from build123d import *

# Parameters (mm, degrees)
SKETCH_1_R           = 3
SKETCH_1_R_2         = 1.2
EXTRUDE_1_DEPTH      = 4.5
EXTRUDE_2_DEPTH      = 4.5
EXTRUDE_2_DEPTH_BACK = 2.5
SKETCH_2_R           = 1.2
FILLET_1_R           = 8
CUT_EXTRUDE_1_REACH  = 62.544
SKETCH_3_R           = 3.421397557
FILLET_2_R           = 3
CUT_EXTRUDE_2_DEPTH  = 1.7
FILLET_START         = 2
FILLET_3_DEPTH       = 2.5


with BuildPart() as part:
    # 草图1 → 凸台-拉伸1 (new body)
    with BuildSketch(Plane.XY):
        Polygon((-12.5, 0), (-18.5, 0), (-18.5, 42.034916596), (0, 60.534916596), (18.5, 42.034916596), (18.5, 0), (12.5, 0), (12.5, 35), (-12.5, 35), align=None)
        with Locations((0, 50.421397557)):
            Circle(SKETCH_1_R, mode=Mode.SUBTRACT)
        with Locations((-15.5, 5)):
            Circle(SKETCH_1_R_2, mode=Mode.SUBTRACT)
        with Locations((-15.5, 26)):
            Circle(SKETCH_1_R_2, mode=Mode.SUBTRACT)
        with Locations(Location((15.5, 5, 0), (0, 0, 180))):
            Circle(SKETCH_1_R_2, mode=Mode.SUBTRACT)
        with Locations(Location((15.5, 26, 0), (0, 0, 180))):
            Circle(SKETCH_1_R_2, mode=Mode.SUBTRACT)
    extrude(amount=EXTRUDE_1_DEPTH)

    # 草图2 → 凸台-拉伸2 (add, two sides: drawn at the far end of the back side and taken through both)
    # profile 1 of 2: a face of its own
    with BuildSketch(Plane.XY.offset(4.5).offset(-EXTRUDE_2_DEPTH_BACK)):
        with BuildLine():
            Line((17.5, 47), (3.906515802, 47))
            ThreePointArc((3.906515802, 47), (5.192959363, 50.421397557), (3.906515802, 53.842795113))
            Line((3.906515802, 53.842795113), (17.5, 53.842795113))
            Line((17.5, 53.842795113), (17.5, 47))
        make_face()
        with Locations(Location((12.5, 50.421397557, 0), (0, 0, 180))):
            Circle(SKETCH_2_R, mode=Mode.SUBTRACT)
    # profile 2 of 2: a face of its own
    with BuildSketch(Plane.XY.offset(4.5).offset(-EXTRUDE_2_DEPTH_BACK)):
        with BuildLine():
            Line((-17.5, 47), (-17.5, 53.842795113))
            Line((-17.5, 53.842795113), (-3.906515802, 53.842795113))
            ThreePointArc((-3.906515802, 53.842795113), (-5.192959363, 50.421397557), (-3.906515802, 47))
            Line((-3.906515802, 47), (-17.5, 47))
        make_face()
        with Locations((-12.5, 50.421397557)):
            Circle(SKETCH_2_R, mode=Mode.SUBTRACT)
    extrude(amount=EXTRUDE_2_DEPTH + EXTRUDE_2_DEPTH_BACK)

    # 圆角1
    fillet_1_edges = [part.edges().sort_by_distance(p)[0] for p in [
        (-18.5, 42.034916596, 2.25),
        (0, 60.534916596, 2.25),
        (18.5, 42.034916596, 2.25),
    ]]
    fillet(fillet_1_edges, radius=FILLET_1_R)

    # 草图3 → 切除-拉伸1 (cut, up to next)
    with BuildSketch(Plane(origin=(0, 0, 2), x_dir=(-1, 0, 0), z_dir=(0, 0, -1)), mode=Mode.PRIVATE) as cut_extrude_1_sk1:
        with Locations((-12.5, 50.421397557)):
            Circle(SKETCH_3_R)
    cut_extrude_1_tool1 = extrude(cut_extrude_1_sk1.sketch, amount=CUT_EXTRUDE_1_REACH, mode=Mode.PRIVATE) & part.part
    # 草图3 → 切除-拉伸1 (cut, up to next)
    with BuildSketch(Plane(origin=(0, 0, 2), x_dir=(-1, 0, 0), z_dir=(0, 0, -1)), mode=Mode.PRIVATE) as cut_extrude_1_sk2:
        with Locations((12.5, 50.421397557)):
            Circle(SKETCH_3_R)
    cut_extrude_1_tool2 = extrude(cut_extrude_1_sk2.sketch, amount=CUT_EXTRUDE_1_REACH, mode=Mode.PRIVATE) & part.part
    add(cut_extrude_1_tool1.solids().sort_by_distance((12.5, 50.421398, 2))[0], mode=Mode.SUBTRACT)
    add(cut_extrude_1_tool2.solids().sort_by_distance((-12.5, 50.421398, 2))[0], mode=Mode.SUBTRACT)

    # 圆角2
    fillet_2_edges = [part.edges().sort_by_distance(p)[0] for p in [
        (9.202203088, 51.332713509, 1),
        (-9.202203088, 51.332713509, 1),
        (-6.692121483, 53.842795113, 3.25),
        (-17.5, 47, 5.5),
        (-5.192959363, 50.421397557, 9),
        (-17.5, 53.842795113, 5.5),
        (6.692121483, 53.842795113, 3.25),
        (17.5, 53.842795113, 5.5),
        (5.192959363, 50.421397557, 9),
        (17.5, 47, 5.5),
    ]]
    fillet(fillet_2_edges, radius=FILLET_2_R)

    # 草图4 → 切除-拉伸2 (cut)
    with BuildSketch(Plane.XY.offset(9)):
        Polygon((0, 46.899022366), (43.079074711, 50.891584803), (0, 53.943772747), (-43.079074711, 50.891584803), align=None)
    extrude(amount=-CUT_EXTRUDE_2_DEPTH, mode=Mode.SUBTRACT)

    # 圆角3: read off the stored shape, not the designer's step
    # 圆角3 outline → 圆角3 (add)
    with BuildSketch(Plane.XY.offset(FILLET_START)):
        with BuildLine():
            ThreePointArc((17.623806552, 42.361452624), (16.757691875, 45.600251323), (17.294803574, 48.909553768))
            ThreePointArc((17.294803574, 48.909553768), (16.192433353, 47.52297167), (14.5, 47))
            Line((14.5, 47), (13.534916596, 47))
            Line((13.534916596, 47), (16.156854249, 44.378062347))
            ThreePointArc((16.156854249, 44.378062347), (16.969389563, 43.42726788), (17.623806552, 42.361452624))
        make_face()
        with BuildLine():
            ThreePointArc((-14.5, 47), (-16.192433353, 47.52297167), (-17.294803574, 48.909553768))
            ThreePointArc((-17.294803574, 48.909553768), (-16.757691875, 45.600251323), (-17.623806552, 42.361452624))
            ThreePointArc((-17.623806552, 42.361452624), (-16.969389563, 43.42726788), (-16.156854249, 44.378062347))
            Line((-16.156854249, 44.378062347), (-13.534916596, 47))
            Line((-13.534916596, 47), (-14.5, 47))
        make_face()
    extrude(amount=FILLET_3_DEPTH)


solid = part.part
CAD build for the part. Positions are in the model's coordinates, mm. A direction names the side the tool comes from. Round coordinates to 2 decimals unless told otherwise and drop trailing zeros. Loops run counter-clockwise (first coordinate to the right, second up) from the corner with the lowest first, then second, coordinate; pieces in that order, holes last.
(1) Cut at C-C (x = 0). Give the cut face in (y, z), plus the area to 3 significant figures.
(2) Which spindle directions (+Z, -Z, +X, -X, +Y, -Y) get a long thin tool onto all of the face, cutting with end or side? Do faces 1 (the flat face through (12.5, 17, 2)), 2 (the cylindrical face through (-10.44, 47.69, 1.01)), 3 (the flat face through (-10, 53.843, 5)), 4 (the flat face through (10.721, 53.184, 8.162)), 5 (the flat face through (-6.948, 53.587, 0.719)). Say none if no direction does.
(3) Cut at B-B (y = 5). Give the cut face in (x, z), plus the area to 3 significant figures.
(4) Two-plate mould, pull along X, no slides. Class faces 6 (the flat face through (-14.803, 45.732, 0.986)), 7 (the flat face through (0.3, 35.4, 0)), 8 (the cylindrical face through (-14.355, 5.36, 2.218)), 9 (the cylindrical face through (0.09, 57.22, 2.28)): +X half, -X half, draft (parallel to the pull), parting line (faces both ways), or undercut.
(5) Cut at D-D (z = 3.5). State how many separate pieces and enclosed holes the cut face has, plus the area to 3 significant figures.
(6) Wall check: line 1 along X through (y, z) = (13, 0.5); line 2 along Y through (x, z) = (15.5, 1.15); line 3 along Z through (x, y) = (3, 48). Give the ranges that are in metal, low to high.
(7) Drop flat-ended pins along their axis: pin 1 (0.9 mm diameter, centred on y = 50.5, z = 4.5, fed in from -X); pin 2 (4 mm diameter, centred on x = -8, z = 7, fed in from -Y); pin 3 (1.3 mm diameter, centred on x = -4, z = 2.5, fed in from -Y); pin 4 (4 mm diameter, centred on x = 11.5, y = 47.5, fed in from -Z). Give the stop position or say it passes through.
(8) Cut at A-A (y = 32.5). Give the cut face in (x, z), plus the area to 3 significant figures.
Findings below:
1. outline: (35, 0) - (47.42, 0) - (47.42, 4.5) - (35, 4.5) - close; (53.42, 0) - (57.22, 0) - (57.22, 4.5) - (53.42, 4.5) - close
1. area: 73.0 mm2
2. face 1: +Z, -Z, -Y
2. face 2: -Z, +Y
2. face 3: +Z, -X, +Y
2. face 4: +Z
2. face 5: -Z, -X, +Y
3. outline: (-18.5, 0) - (-16.7, 0) - (-16.7, 4.5) - (-18.5, 4.5) - close; (-14.3, 0) - (-12.5, 0) - (-12.5, 4.5) - (-14.3, 4.5) - close; (12.5, 0) - (14.3, 0) - (14.3, 4.5) - (12.5, 4.5) - close; (16.7, 0) - (18.5, 0) - (18.5, 4.5) - (16.7, 4.5) - close
3. area: 32.4 mm2
4. face 6: -X half
4. face 7: draft
4. face 8: undercut
4. face 9: parting line
5. separate pieces: 1
5. enclosed holes: 7
5. area: 1,060 mm2
6. line 1: x = -18.5 to -12.5, 12.5 to 18.5
6. line 2: y = 0 to 3.8, 6.2 to 24.8, 27.2 to 45.03
6. line 3: z = 0 to 4.5
7. pin 1: stops at x = -17.5
7. pin 2: stops at y = 47
7. pin 3: stops at y = 35
7. pin 4: stops at z = 0
8. outline: (-18.5, 0) - (-12.5, 0) - (-12.5, 4.5) - (-18.5, 4.5) - close; (12.5, 0) - (18.5, 0) - (18.5, 4.5) - (12.5, 4.5) - close
8. area: 54.0 mm2
